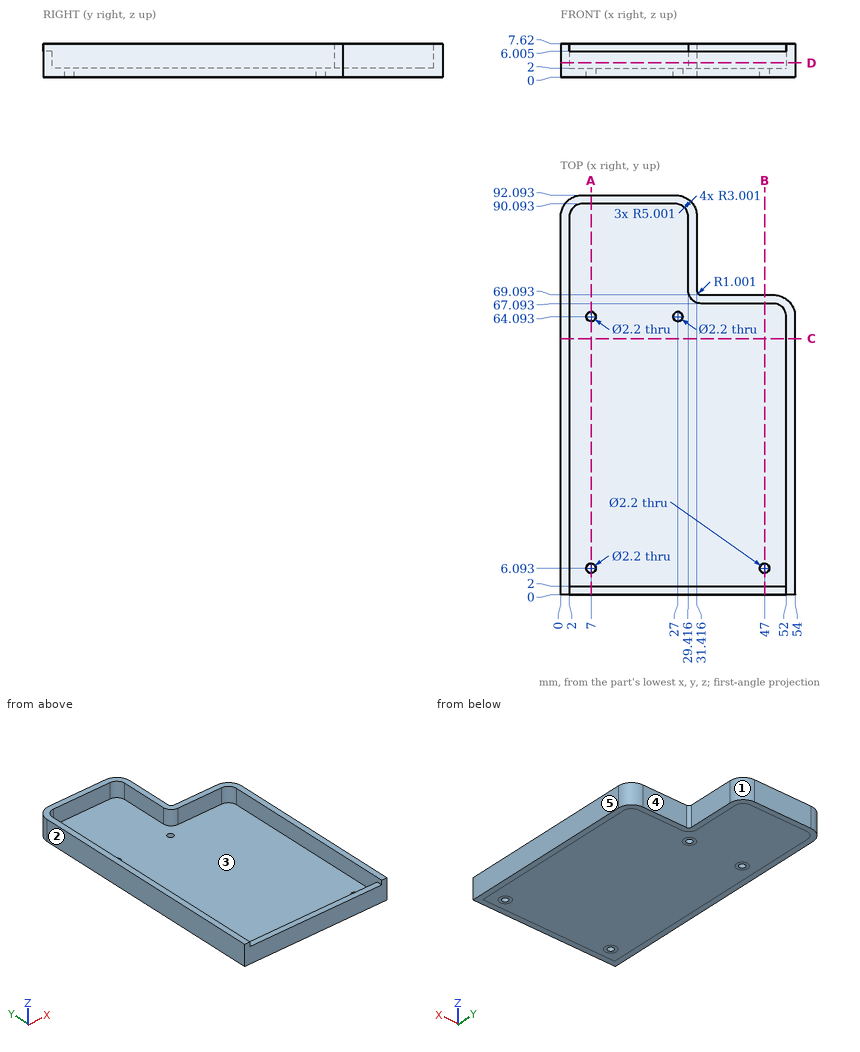
The figure shows three views and two pictorial views of one solid part (mm, origin at its lowest corner). Answer the questions. A direction names the side the tool comes from. Round coordinates to 2 decimals unless told otherwise and drop trailing zeros. Loops run counter-clockwise (first coordinate to the right, second up) from the corner with the lowest first, then second, coordinate; pieces in that order, holes last. Notation, with made-up numbers: (-7, 6.25) - (4, 6.25) arc R21 cw to (4, 10.25) - close; hole circle Ø11 at (80, 31.5). An arc over 180 degrees is marked (long way). One line per question, with ' | ' between items. Start each with the question number.
Q1. Flat-ended cylindrical pins translate along their axes: pin 1 (3.5 mm diameter, centred on x = 7, y = 64.09, fed in from +Z); pin 2 (4 mm diameter, centred on x = 13.5, y = 63.5, fed in from -Z); pin 3 (1.8 mm diameter, centred on x = 7, y = 6.09, fed in from -Z); pin 4 (4 mm diameter, centred on y = 81.5, z = 4, fed in from +X). Find the tip coordinate at first contact, or state that the pin passes through.
Q2. For the marked faces 4 and 5, determine the directions among +Z, -Z, +X, -X, +Y, -Y from which every point of the face is accessible in a straight line to the end or side of a thin tool.
Q3. Section D-D on z = 3.25 is taken. Give the vertices of the cut face in (x, y) (1 decimal).
Q4. Section A-A on x = 7 is taken. Give the vertices of the cut face in (y, z) (1 decimal).
Q5. Find the intervals of material crossed by L1, parallel to Y at x = 7, z = 1; L2, parallel to X at y = 43, z = 2.5; L3, parallel to Y at x = 47, z = 1.15, in increasing order.
Q6. Section B-B on x = 47 is taken. Give the vertices of the cut face in (y, z) (1 decimal).
Q7. Section C-C on y = 59 is taken. Give the vertices of the cut face in (x, z).
Q8. For a pull along X with two mould halves and no side action, classify the marked faces 1, 2 and 3 as +X half, -X half, draft (parallel to the pull), parting line (faces both ways), or undercut.
Established:
1) pin 1: z = 2 | pin 2: z = 0 | pin 3: through | pin 4: x = 31.42
2) face 4: +Z, -Z, +X, +Y | face 5: +Z, -Z, +X, +Y, -Y
3) outline: (0, 0) - (54, 0) - (54, 64.1) arc R5 ccw to (49, 69.1) - (32.4, 69.1) arc R1 cw to (31.4, 70.1) - (31.4, 87.1) arc R5 ccw to (26.4, 92.1) - (5, 92.1) arc R5 ccw to (0, 87.1) - close; hole (2, 2) - (52, 2) - (52, 64.1) arc R3 ccw to (49, 67.1) - (32.4, 67.1) arc R3 cw to (29.4, 70.1) - (29.4, 87.1) arc R3 ccw to (26.4, 90.1) - (5, 90.1) arc R3 ccw to (2, 87.1) - close
4) outline: (0, 0) - (5, 0) - (5, 2) - (2, 2) - (2, 6) - (0, 6) - close; (7.2, 0) - (63, 0) - (63, 2) - (7.2, 2) - close; (65.2, 0) - (92.1, 0) - (92.1, 7.6) - (90.1, 7.6) - (90.1, 2) - (65.2, 2) - close
5) L1: 0 to 4.99, 7.19 to 62.99, 65.19 to 92.09 | L2: 0 to 2, 52 to 54 | L3: 0 to 4.99, 7.19 to 69.09
6) outline: (0, 0) - (5, 0) - (5, 2) - (2, 2) - (2, 6) - (0, 6) - close; (7.2, 0) - (69.1, 0) - (69.1, 7.6) - (67.1, 7.6) - (67.1, 2) - (7.2, 2) - close
7) outline: (0, 0) - (54, 0) - (54, 7.62) - (52, 7.62) - (52, 2) - (2, 2) - (2, 7.62) - (0, 7.62) - close
8) face 1: +X half | face 2: -X half | face 3: undercut
